Design review of the part built by this model. Coordinates are the model's own, in mm. Face numbers are marked on the shaded views. A direction names the side the tool comes from. Give positions to 0.01 mm unless a question says otherwise; leave off trailing zeros. Order: outer loops, then holes, each group sorted by start corner. A loop starts at its lowest first (then second) coordinate and runs counter-clockwise, first axis right, second up. Notation, with made-up numbers: M 11,-23.75 L 16,-23.75 A11 ccw 16,-19.75 Z; hole C -13,31.25 d5. An arc over 180 degrees is marked long. Answer as a JSON object with one key per item and string values.
Autodesk Inventor part; units mm, degrees
ref_plane "YZ Plane" through (0, 0, 0) normal (1, 0, 0) x (0, 1, 0)
ref_plane "XZ Plane" through (0, 0, 0) normal (0, 1, 0) x (-1, 0, 0)
ref_plane "XY Plane" through (0, 0, 0) normal (0, 0, 1) x (1, 0, 0)
sketch "Sketch1" plane through (0, 0, 0) normal (0, 0, 1) x (1, 0, 0)
  line L0 (0, 0) -> (2, 0)
  line L1 (2, 0) -> (2, 16)
  line L2 (2, 16) -> (0, 16)
  line L3 (0, 16) -> (0, 0)
  line L4 (2, 2) -> (11, 2)
  line L5 (11, 2) -> (11, 0)
  line L6 (11, 0) -> (2, 0)
  line L7 (2, 0) -> (2, 2)
  dimension "d0" = 2
  dimension "d1" = 16
  dimension "d2" = 9
extrude "Extrusion1" add sketch "Sketch1" against normal blind 22
sketch "Sketch3" plane through (2, 2, 0) normal (1, 0, 0) x (0, 0, -1)
  line L0 (9.5, 14) -> (4.5, 14)
  line L1 (4.5, 14) -> (4.5, 8)
  line L2 (4.5, 8) -> (9.5, 8)
  line L3 (9.5, 8) -> (9.5, 14)
  point P0 (0, -2)
  dimension "d9" = 5
  dimension "d10" = 6
extrude "Extrusion3" cut sketch "Sketch3" against normal blind 10
fillet "Fillet1" radius 0.8 7 edges at (2, 10, -7) (0, 10, -7) (1, 16, -9.5) (2, 13, -9.5) (0, 13, -9.5) (2, 13, -4.5) (0, 13, -4.5)
properties part number "housing_mate_v08"
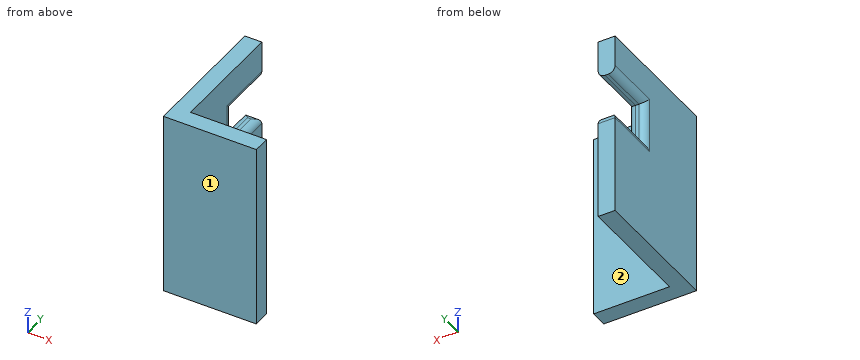
(1) We need section D-D (z = -12.75). Write out the cut boundary in (x, y), plus the area to 3 significant figures.
Checked values:
{"outline": "M 0,0 L 11,0 L 11,2 L 2,2 L 2,16 L 0,16 Z", "area": "50.0 mm^2"}
(2) We need section A-A (y = 12.25). Write out the cut boundary in (x, z), plus the area to 3 significant figures.
Checked values:
{"outline": "M 0,-22 L 2,-22 L 2,-10.3 A0.8 ccw 1.2,-9.5 L 0.8,-9.5 A0.8 ccw 0,-10.3 Z; M 0,-3.7 A0.8 ccw 0.8,-4.5 L 1.2,-4.5 A0.8 ccw 2,-3.7 L 2,0 L 0,0 Z", "area": "33.5 mm^2"}
(3) Tool access review of the marked faces 1 and 2: name each direction out of +Z, -Z, +X, -X, +Y, -Y from which nothing blocks a thin tool from reaching the whole face with its end or side.
Checked values:
{"face 1": "+Z, -Z, +X, -X, -Y", "face 2": "+Z, -Z, +X, +Y"}
(4) We need section B-B (z = -5.75). Write out the cut boundary in (x, y), plus the area to 3 significant figures.
Checked values:
{"outline": "M 0,0 L 11,0 L 11,2 L 2,2 L 2,9.2 A0.8 ccw 1.2,10 L 0.8,10 A0.8 ccw 0,9.2 Z", "area": "37.7 mm^2"}
(5) We need section C-C (x = 1.5). Write out the cut boundary in (y, z).
Checked values:
{"outline": "M 0,-22 L 16,-22 L 16,-10.3 A0.8 ccw 15.5,-9.56 L 9.94,-9.56 L 9.94,-4.44 L 16,-4.44 L 16,0 L 0,0 Z"}
(6) To check wall thickness, follow L1, parallel to X at y = 14, z = -12.25; L2, parallel to Z at x = 0.5, y = 14.25. State the ranges of each line that lie inside material, in increasing order. Write a range as from..to.
Checked values:
{"L1": "x = 0..2", "L2": "z = -22..-9.56, -4.44..0"}
(7) Insertion check: pin 1 (4 mm diameter, centred on y = 4.5, z = -4, fed in from +X); pin 2 (6 mm diameter, centred on x = 2.5, z = -7.5, fed in from +Y); pin 3 (3 mm diameter, centred on x = 9, z = -14, fed in from +Y). Each pin has a flat end and moves straight along its axis. Give the tip position at first contact, or say it passes through.
Checked values:
{"pin 1": "stops at x = 2", "pin 2": "stops at y = 16", "pin 3": "stops at y = 2"}
